```python
from build123d import *

# Parameters (mm, degrees)
BOSS_EXTRUDE1_DEPTH = 292.1
FILLET1_R           = 0.79375
FILLET2_R           = 2.3495


with BuildPart() as part:
    # Sketch1 → Boss-Extrude1 (new body)
    with BuildSketch(Plane.XY):
        Polygon((-17.4625, 11.1125), (-17.4625, 0), (17.4625, 0), (17.4625, 11.1125), (15.08125, 11.1125), (15.08125, 9.525), (15.875, 9.525), (15.875, 1.5875), (-15.875, 1.5875), (-15.875, 9.525), (-15.08125, 9.525), (-15.08125, 11.1125), align=None)
    extrude(amount=BOSS_EXTRUDE1_DEPTH)

    # Fillet1
    fillet1_edges = [part.edges().sort_by_distance(p)[0] for p in [
        (15.875, 1.5875, 146.05),
        (-15.875, 1.5875, 146.05),
        (-15.08125, 9.525, 146.05),
        (-15.08125, 11.1125, 146.05),
        (-17.4625, 11.1125, 146.05),
        (17.4625, 11.1125, 146.05),
        (15.08125, 11.1125, 146.05),
        (15.08125, 9.525, 146.05),
    ]]
    fillet(fillet1_edges, radius=FILLET1_R - 0.0001)  # a hair under: the kernel refuses the full size

    # Fillet2
    fillet2_edges = [part.edges().sort_by_distance(p)[0] for p in [
        (17.4625, 0, 146.05),
        (-17.4625, 0, 146.05),
    ]]
    fillet(fillet2_edges, radius=FILLET2_R)


solid = part.part
```
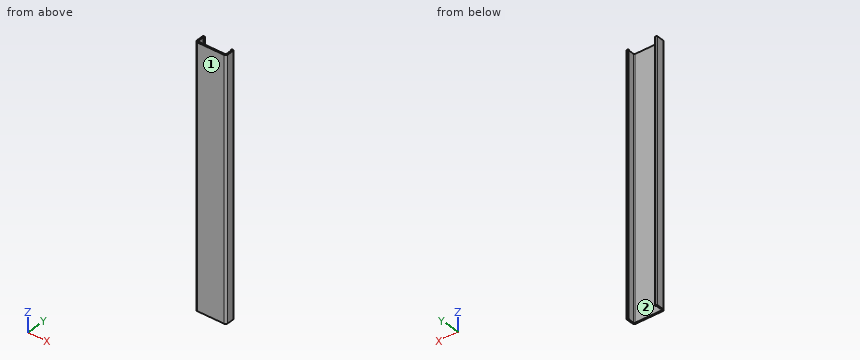
Geometry: final body of the model. Coordinates: model frame, mm. Face numbers are marked on the shaded views. Round coordinates to 2 decimals unless told otherwise and drop trailing zeros. Order: outer loops, then holes, each group sorted by start corner. A loop starts at its lowest first (then second) coordinate and runs counter-clockwise, first axis right, second up. Notation, with made-up numbers: (23, 85.25) - (29, 85.25) arc R34 cw to (29, 119.25) - close; hole circle Ø6 at (66.5, 40.25). An arc over 180 degrees is marked (long way). Write item = value, one per line. Start each with the question number.
Q1. Cut plane A-A on y = 5.75. Return the cut outline in (x, z) (1 decimal), and give its area (3 significant figures).
Q2. Pin query (flat end, axial travel): pin 1 (5 mm diameter, centred on x = 7, y = 5.5, fed in from -Z); pin 2 (9 mm diameter, centred on x = -6.5, z = 92.5, fed in from +Y). Return the tip coordinate at first contact, or that it passes through.
Q3. Cut plane C-C on x = 4.5. Return the cut outline in (y, z).
Q4. Pull-direction query (X, two-part tool) for the marked faces 1 and 2; classes: +X half, -X half, draft (parallel to the pull), parting line (faces both ways), or undercut.
Q5. Ray query, line 1 (X direction, y = 8.5, z = 105.5) (1 decimal); line 2 (Y direction, x = -15, z = 254). Return the intervals inside material, ascending. Write a range as from..to.
Outcome:
q1.outline = (-17.5, 0) - (-15.9, 0) - (-15.9, 292.1) - (-17.5, 292.1) - close; (15.9, 0) - (17.5, 0) - (17.5, 292.1) - (15.9, 292.1) - close
q1.area = 927 mm^2
q2.pin_1 = through
q2.pin_2 = 1.59
q3.outline = (0, 0) - (1.59, 0) - (1.59, 292.1) - (0, 292.1) - close
q4.face_1 = draft
q4.face_2 = undercut
q5.line_1 = -17.5..-15.9, 15.9..17.5
q5.line_2 = 0..1.59
